from build123d import *

# Parameters (mm, degrees)
ESBO_O1_R                = 3
RESSALTO_EXTRUS_O1_DEPTH = 8
ESBO_O2_R                = 5
ESBO_O2_R_2              = 3
RESSALTO_EXTRUS_O2_DEPTH = 1
ESBO_O3_R                = 6
ESBO_O3_R_2              = 3
RESSALTO_EXTRUS_O3_DEPTH = 20


with BuildPart() as part:
    # Esboço1 → Ressalto-extrusão1 (new body)
    with BuildSketch(Plane.XY):
        Polygon((-8.660254038, 5), (-8.660254038, -5), (0, -10), (8.660254038, -5), (8.660254038, 5), (0, 10), align=None)
        Circle(ESBO_O1_R, mode=Mode.SUBTRACT)
    extrude(amount=RESSALTO_EXTRUS_O1_DEPTH)

    # Esboço2 → Ressalto-extrusão2 (add)
    with BuildSketch(Plane(origin=(0, 0, 0), x_dir=(-1, 0, 0), z_dir=(0, 0, -1))):
        Circle(ESBO_O2_R)
        Circle(ESBO_O2_R_2, mode=Mode.SUBTRACT)
    extrude(amount=RESSALTO_EXTRUS_O2_DEPTH)

    # Esboço3 → Ressalto-extrusão3 (add)
    with BuildSketch(Plane.XY.offset(8)):
        Circle(ESBO_O3_R)
        Circle(ESBO_O3_R_2, mode=Mode.SUBTRACT)
    extrude(amount=RESSALTO_EXTRUS_O3_DEPTH)


solid = part.part
Geometry check sheet. Reference: the model listing, model coordinates, mm. A direction names the side the tool comes from. Round coordinates to 2 decimals unless told otherwise and drop trailing zeros. Write each loop counter-clockwise with the first axis right and the second up, starting at its lowest first coordinate (ties: lowest second). Pieces come first, ordered by that corner, then holes. Notation, with made-up numbers: (-11.5, 65) -> (30.5, 65) arc R33 cw to (30.5, 99) -> close; hole circle Ø5 at (33, -32.5). An arc over 180 degrees is marked (long way). One line per item, written item: value. Start each with the question number.
(1) Cross-section at B-B, the plane z = 2.75. Record the cut outline in (x, y).
(2) Access from +Z, -Z, +X, -X, +Y, -Y to the whole of each face (thin tool, end or side, straight path). Record for faces 1 (the flat face through (8.66, 0, 4)), 2 (the cylindrical face through (1.08, -4.88, -0.49)), 3 (the cylindrical face through (-6, 0, 18)).
(3) Scan lines: line 1 (Y direction, x = 0, z = 14.5); line 2 (X direction, y = 0, z = 5.25); line 3 (Y direction, x = 0, z = -0.5). Record each from-to range of solid material in increasing order. Write a range as [from, to].
(4) Cross-section at D-D, the plane x = 6.5. Record the cut outline in (y, z).
(5) Cross-section at A-A, the plane y = 0. Record the cut outline in (x, z).
(6) Go/stop test with flat-tipped pins: pin 1 Ø5 at (x, z) = (-6.5, 6.5) entering from -Y; pin 2 Ø8 at (y, z) = (4.5, 15) entering from +X; pin 3 Ø5 at (y, z) = (2.5, 24.5) entering from -X. Record where each tip stops, or that it passes through.
(7) Cross-section at C-C, the plane x = 1.75. Record the cut outline in (y, z), and give its area (3 significant figures).
Answer:
1. outline: (-8.66, -5) -> (0, -10) -> (8.66, -5) -> (8.66, 5) -> (0, 10) -> (-8.66, 5) -> close; hole circle Ø6 at (0, 0)
2. face 1: +Z, -Z, +X, +Y, -Y
2. face 2: -Z
2. face 3: +Z
3. line 1: [-6, -3], [3, 6]
3. line 2: [-8.66, -3], [3, 8.66]
3. line 3: [-5, -3], [3, 5]
4. outline: (-6.25, 0) -> (6.25, 0) -> (6.25, 8) -> (-6.25, 8) -> close
5. outline: (-8.66, 0) -> (-5, 0) -> (-5, -1) -> (-3, -1) -> (-3, 28) -> (-6, 28) -> (-6, 8) -> (-8.66, 8) -> close; (3, -1) -> (5, -1) -> (5, 0) -> (8.66, 0) -> (8.66, 8) -> (6, 8) -> (6, 28) -> (3, 28) -> close
6. pin 1: y = -7.69
6. pin 2: x = 5.98
6. pin 3: x = -6
7. outline: (-8.99, 0) -> (-4.68, 0) -> (-4.68, -1) -> (-2.44, -1) -> (-2.44, 28) -> (-5.74, 28) -> (-5.74, 8) -> (-8.99, 8) -> close; (2.44, -1) -> (4.68, -1) -> (4.68, 0) -> (8.99, 0) -> (8.99, 8) -> (5.74, 8) -> (5.74, 28) -> (2.44, 28) -> close
7. area: 241 mm²
